CAD build for the part. Positions are in the model's coordinates, mm. Coordinates: 2 decimals unless noted, no trailing zeros. Loops run counter-clockwise (first coordinate to the right, second up) from the corner with the lowest first, then second, coordinate; pieces in that order, holes last. Notation, with made-up numbers: (24, 28.5) -> (70, 28.5) arc R23 ccw to (70, 48.5) -> close; hole circle Ø5 at (-24.75, 58.5). An arc over 180 degrees is marked (long way). Write each question's results on one line, items separated by ' | '.
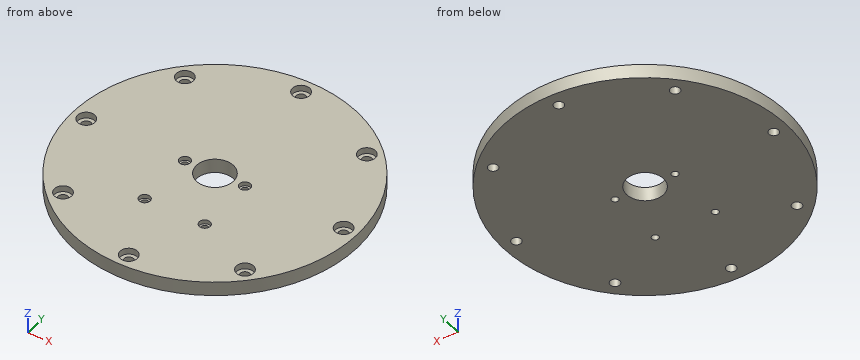
```python
from build123d import *

# Parameters (mm, degrees)
SKETCH_1_R                   = 50
EXTRUDE_1_DEPTH              = 5
HOLE_WIZARD_M2_1_D           = 2.4
HOLE_WIZARD_M2_1_CBORE_D     = 3.85
HOLE_WIZARD_M2_1_CBORE_DEPTH = 1.45
HOLE_WIZARD_M3_2_D           = 3.4
HOLE_WIZARD_M3_2_CBORE_D     = 6.05
HOLE_WIZARD_M3_2_CBORE_DEPTH = 2.2
PATTERN_CIRCULAR_1_COUNT     = 8
SKETCH_6_R                   = 6.5
CUT_EXTRUDE_1_DEPTH          = 71.887234394


with BuildPart() as part:
    # ｽｹｯﾁ1 → ﾎﾞｽ - 押し出し1 (new body)
    with BuildSketch(Plane.XY):
        Circle(SKETCH_1_R)
    extrude(amount=EXTRUDE_1_DEPTH)

    # M2 丸平ねじ用座ぐり穴1 (through all)
    with Locations(Plane.XY.offset(5)):
        with Locations((-10.5, 0), (-10.5, -21)):
            hole_wizard_m2_1 = CounterBoreHole(HOLE_WIZARD_M2_1_D / 2, HOLE_WIZARD_M2_1_CBORE_D / 2, HOLE_WIZARD_M2_1_CBORE_DEPTH)

    # ﾐﾗｰ1: M2 丸平ねじ用座ぐり穴1 across plane
    add(hole_wizard_m2_1.mirror(Plane(origin=(0, 0, 0), x_dir=(0, 0, 1), z_dir=(1, 0, 0))), mode=Mode.SUBTRACT)

    # M3 丸平ねじ用座ぐり穴2 (through all)
    with Locations(Plane.XY.offset(5)):
        with Locations((45, 0)):
            hole_wizard_m3_2 = CounterBoreHole(HOLE_WIZARD_M3_2_D / 2, HOLE_WIZARD_M3_2_CBORE_D / 2, HOLE_WIZARD_M3_2_CBORE_DEPTH)

    # 円形ﾊﾟﾀｰﾝ1: M3 丸平ねじ用座ぐり穴2 ×8 about axis
    pattern_circular_1_axis = Axis((0, 0, 0), (0, 0, 1))
    for i in range(1, PATTERN_CIRCULAR_1_COUNT):
        add(hole_wizard_m3_2.rotate(pattern_circular_1_axis, i * 360 / PATTERN_CIRCULAR_1_COUNT), mode=Mode.SUBTRACT)

    # ｽｹｯﾁ6 → ｶｯﾄ - 押し出し1 (cut, through all)
    with BuildSketch(Plane.XY.offset(5)):
        Circle(SKETCH_6_R)
    extrude(amount=-CUT_EXTRUDE_1_DEPTH, mode=Mode.SUBTRACT)


solid = part.part
```
Q1. Cut at B-B on y = -5. Write the cut outline in (x, z), and give its area (3 significant figures).
Results are:
outline: (-49.75, 0) -> (-4.15, 0) -> (-4.15, 5) -> (-49.75, 5) -> close; (4.15, 0) -> (49.75, 0) -> (49.75, 5) -> (4.15, 5) -> close | area: 456 mm^2
Q2. Cut at A-A on x = 0. Write the cut outline in (y, z) (3 decimals), and give its area (3 significant figures).
Results are:
outline: (-50, 0) -> (-46.7, 0) -> (-46.7, 2.8) -> (-48.025, 2.8) -> (-48.025, 5) -> (-50, 5) -> close; (-43.3, 0) -> (-6.5, 0) -> (-6.5, 5) -> (-41.975, 5) -> (-41.975, 2.8) -> (-43.3, 2.8) -> close; (6.5, 0) -> (43.3, 0) -> (43.3, 2.8) -> (41.975, 2.8) -> (41.975, 5) -> (6.5, 5) -> close; (46.7, 0) -> (50, 0) -> (50, 5) -> (48.025, 5) -> (48.025, 2.8) -> (46.7, 2.8) -> close | area: 389 mm^2
Q3. Cut at C-C on z = 1.2. Give the number of separate pieces and of enclosed holes in the cut face, and give its area (3 significant figures).
Results are:
separate pieces: 1 | enclosed holes: 13 | area: 7,630 mm^2
Q4. Drop flat-ended pins along their axis: pin 1 (5.5 mm diameter, centred on x = 31.82, y = 31.82, fed in from +Z); pin 2 (2 mm diameter, centred on y = -22.5, z = 3, fed in from -X); pin 3 (1.9 mm diameter, centred on x = 11, y = 0.5, fed in from +Z). Give the stop position or say it passes through.
Results are:
pin 1: z = 2.8 | pin 2: x = -45.14 | pin 3: z = 3.55
Q5. Wall check: L1, parallel to Y at x = -10.5, z = 0.95; L2, parallel to Y at x = -1, z = 1.1; L3, parallel to Y at x = -34.5, z = 3.4. Give the ranges that are in metal, low to high. Write a range as from..to.
Results are:
L1: -48.89..-22.2, -19.8..-1.2, 1.2..48.89 | L2: -49.99..-46.37, -43.63..-6.42, 6.42..43.63, 46.37..49.99 | L3: -36.19..-33.22, -30.42..30.42, 33.22..36.19
Q6. Cut at D-D on y = -21. Write the cut outline in (x, z) (3 decimals), and give its area (3 significant figures).
Results are:
outline: (-45.376, 0) -> (-11.7, 0) -> (-11.7, 3.55) -> (-12.425, 3.55) -> (-12.425, 5) -> (-45.376, 5) -> close; (-9.3, 0) -> (9.3, 0) -> (9.3, 3.55) -> (8.575, 3.55) -> (8.575, 5) -> (-8.575, 5) -> (-8.575, 3.55) -> (-9.3, 3.55) -> close; (11.7, 0) -> (45.376, 0) -> (45.376, 5) -> (12.425, 5) -> (12.425, 3.55) -> (11.7, 3.55) -> close | area: 426 mm^2
